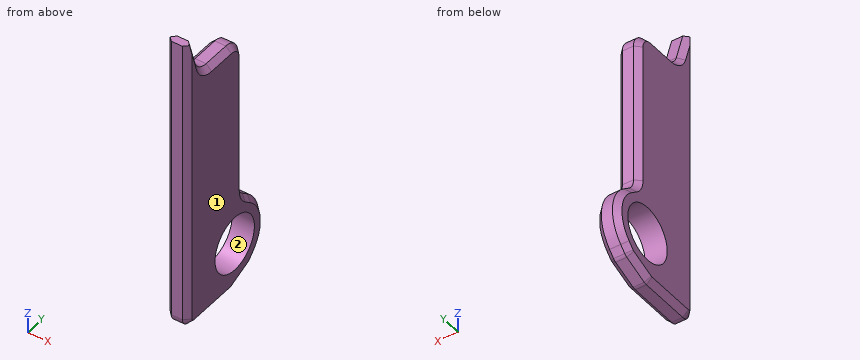
```python
from build123d import *

# Parameters (mm, degrees)
SKETCH_1_R      = 50
EXTRUDE_1_DEPTH = 40
FILLET_1_R      = 15
FILLET_2_R      = 15
CHAMFER_1_SIZE  = 10


with BuildPart() as part:
    # 草图1 → 凸台-拉伸1 (new body)
    with BuildSketch(Plane(origin=(0, 0, 0), x_dir=(0, 0, -1), z_dir=(1, 0, 0))):
        with BuildLine():
            Line((85, -8.5), (65, 41.5))
            Line((65, 41.5), (52.08314884, 53.966152419))
            ThreePointArc((52.08314884, 53.966152419), (-5.26193851, 74.815185645), (-59.124192044, 46.14466291))
            Line((-59.124192044, 46.14466291), (-69.350323182, 33.042134836))
            ThreePointArc((-69.350323182, 33.042134836), (-79.842035775, 24.539510808), (-93, 21.5))
            Line((-93, 21.5), (-348, 21.5))
            ThreePointArc((-348, 21.5), (-369.213203436, 12.713203436), (-378, -8.5))
            Line((-378, -8.5), (-378, -58.5))
            ThreePointArc((-378, -58.5), (-383.833102889, -76.275294204), (-399.064072268, -87.138247076))
            Line((-399.064072268, -87.138247076), (-451.500924593, -103.5))
            Line((-451.500924593, -103.5), (-451.500924593, -118.5))
            Line((-451.500924593, -118.5), (-116.500924593, -118.5))
            Line((-116.500924593, -118.5), (85, -118.5))
            Line((85, -118.5), (85, -8.5))
        make_face()
        Circle(SKETCH_1_R, mode=Mode.SUBTRACT)
    extrude(amount=EXTRUDE_1_DEPTH)

    # 圆角1
    fillet_1_edges = [part.edges().sort_by_distance(p)[0] for p in [
        (20, -118.5, -85),
    ]]
    fillet(fillet_1_edges, radius=FILLET_1_R)

    # 圆角2
    fillet_2_edges = [part.edges().sort_by_distance(p)[0] for p in [
        (20, 41.5, -65),
        (20, -8.5, -85),
    ]]
    fillet(fillet_2_edges, radius=FILLET_2_R)

    # 倒角1
    # the kernel refuses this chamfer: 10 mm, written as the material it takes off along each edge
    with BuildSketch(Plane(origin=(40, -118.5, -70), x_dir=(0.027495876610586317, 0.9996219169112968, 0), z_dir=(0, 0, 1))) as chamfer_1_piece_1:
        Polygon((CHAMFER_1_SIZE * 0.999621916911, CHAMFER_1_SIZE * 0.0274958766106), (-CHAMFER_1_SIZE * 0.0274958766106, CHAMFER_1_SIZE * 0.999621916911), (0, 0), align=None)
    extrude(amount=547.217754472, mode=Mode.SUBTRACT)
    with BuildSketch(Plane(origin=(0, -118.5, 477.217754472), x_dir=(0.9996219169112968, -0.027495876610586317, 0), z_dir=(0, 0, -1))) as chamfer_1_piece_2:
        Polygon((CHAMFER_1_SIZE * 0.999621916911, -CHAMFER_1_SIZE * 0.0274958766106), (-CHAMFER_1_SIZE * 0.0274958766106, -CHAMFER_1_SIZE * 0.999621916911), (0, 0), align=None)
    extrude(amount=547.217754472, mode=Mode.SUBTRACT)
    with BuildSketch(Plane(origin=(40, -87.138247076, 399.064072268), x_dir=(0.02749587661058635, -0.9542473146313191, -0.2977516402781551), z_dir=(0, -0.297864257716727, 0.9546082358616352)), Plane(origin=(0, -87.138247076, 399.064072268), x_dir=(0.9996219169112968, 0.026247790264700862, 0.008190038876882964), z_dir=(0, -0.297864257716727, 0.9546082358616352))) as chamfer_1_piece_3:
        Polygon((CHAMFER_1_SIZE * 0.999621916911, -CHAMFER_1_SIZE * 0.0274958766106), (-CHAMFER_1_SIZE * 0.0274958766106, -CHAMFER_1_SIZE * 0.999621916911), (0, 0), align=None)
    extrude(amount=80.647062361, mode=Mode.SUBTRACT)
    with BuildSketch(Plane(origin=(40, -58.5, 408), x_dir=(0, 0, -1), z_dir=(0, 1, 0))) as chamfer_1_piece_4:
        Polygon((30 + CHAMFER_1_SIZE, 0), (30, CHAMFER_1_SIZE), (30, 0), align=None)
    revolve(axis=Axis((40, -58.5, 408), (-1, 0, 0)), revolution_arc=72.670629443, mode=Mode.SUBTRACT)
    with BuildSketch(Plane(origin=(40, -8.5, 378), x_dir=(0.027495876610586282, 0, -0.9996219169112968), z_dir=(0, -1, 0)), Plane(origin=(0, -8.5, 378), x_dir=(0.9996219169112968, 0, 0.0274958766105877), z_dir=(0, -1, 0))) as chamfer_1_piece_5:
        Polygon((CHAMFER_1_SIZE * 0.999621916911, -CHAMFER_1_SIZE * 0.0274958766106), (-CHAMFER_1_SIZE * 0.0274958766106, -CHAMFER_1_SIZE * 0.999621916911), (0, 0), align=None)
    extrude(amount=50, mode=Mode.SUBTRACT)
    with BuildSketch(Plane(origin=(40, -8.5, 348), x_dir=(0, 1, 0), z_dir=(0, 0, -1))) as chamfer_1_piece_6:
        Polygon((30 - CHAMFER_1_SIZE, 0), (30, -CHAMFER_1_SIZE), (30, 0), align=None)
    revolve(axis=Axis((40, -8.5, 348), (1, 0, 0)), revolution_arc=90, mode=Mode.SUBTRACT)
    with BuildSketch(Plane(origin=(40, 21.5, 93), x_dir=(0.027495876610586317, -0.9996219169112968, 0), z_dir=(0, 0, 1)), Plane(origin=(0, 21.5, 93), x_dir=(0.9996219169112968, 0.027495876610586317, 0), z_dir=(0, 0, 1))) as chamfer_1_piece_7:
        Polygon((CHAMFER_1_SIZE * 0.999621916911, -CHAMFER_1_SIZE * 0.0274958766106), (-CHAMFER_1_SIZE * 0.0274958766106, -CHAMFER_1_SIZE * 0.999621916911), (0, 0), align=None)
    extrude(amount=255, mode=Mode.SUBTRACT)
    with BuildSketch(Plane(origin=(40, 51.5, 93), x_dir=(0, -0.6152621721387623, -0.7883225605899479), z_dir=(0, 0.7883225605899479, -0.6152621721387623))) as chamfer_1_piece_8:
        Polygon((30 + CHAMFER_1_SIZE, 0), (30, CHAMFER_1_SIZE), (30, 0), align=None)
    revolve(axis=Axis((40, 51.5, 93), (-1, 0, 0)), revolution_arc=52.029027347, mode=Mode.SUBTRACT)
    with BuildSketch(Plane(origin=(40, 46.14466291, 59.124192044), x_dir=(0.027495876610586327, -0.6150295519163572, -0.788024509161346), z_dir=(0, -0.7883225605899483, 0.6152621721387617)), Plane(origin=(0, 46.14466291, 59.124192044), x_dir=(0.9996219169112968, 0.016917172768288757, 0.021675619855322733), z_dir=(0, -0.7883225605899483, 0.6152621721387617))) as chamfer_1_piece_9:
        Polygon((CHAMFER_1_SIZE * 0.999621916911, -CHAMFER_1_SIZE * 0.0274958766106), (-CHAMFER_1_SIZE * 0.0274958766106, -CHAMFER_1_SIZE * 0.999621916911), (0, 0), align=None)
    extrude(amount=16.620770139, mode=Mode.SUBTRACT)
    with BuildSketch(Plane(origin=(40, 0, 0), x_dir=(0, 0.7195486989139618, -0.6944419845395472), z_dir=(0, -0.6944419845395472, -0.7195486989139618))) as chamfer_1_piece_10:
        Polygon((75 - CHAMFER_1_SIZE, 0), (75, -CHAMFER_1_SIZE), (75, 0), align=None)
    revolve(axis=Axis((40, 0, 0), (1, 0, 0)), revolution_arc=96.011794601, mode=Mode.SUBTRACT)
    with BuildSketch(Plane(origin=(40, 43.734636446, -62.684572962), x_dir=(0.027495876610586317, -0.7192766497194039, 0.6941794277691075), z_dir=(0, 0.6944419845395474, 0.7195486989139617)), Plane(origin=(0, 43.734636446, -62.684572962), x_dir=(0.9996219169112968, 0.019784622240646275, -0.019094291120110143), z_dir=(0, 0.6944419845395474, 0.7195486989139617))) as chamfer_1_piece_11:
        Polygon((CHAMFER_1_SIZE * 0.999621916911, -CHAMFER_1_SIZE * 0.0274958766106), (-CHAMFER_1_SIZE * 0.0274958766106, -CHAMFER_1_SIZE * 0.999621916911), (0, 0), align=None)
    extrude(amount=14.733435189, mode=Mode.SUBTRACT)
    with BuildSketch(Plane(origin=(40, 32.941405963, -52.267943193), x_dir=(0, 0.3713906763541047, -0.9284766908852589), z_dir=(0, -0.9284766908852589, -0.3713906763541047))) as chamfer_1_piece_12:
        Polygon((15 - CHAMFER_1_SIZE, 0), (15, -CHAMFER_1_SIZE), (15, 0), align=None)
    revolve(axis=Axis((40, 32.941405963, -52.267943193), (1, 0, 0)), revolution_arc=24.215823259, mode=Mode.SUBTRACT)
    with BuildSketch(Plane(origin=(40, -5.817875908, -83.927150363), x_dir=(0.027495876610586313, -0.37125025982007287, 0.9281256495501801), z_dir=(0, 0.9284766908852591, 0.37139067635410444)), Plane(origin=(0, -5.817875908, -83.927150363), x_dir=(0.9996219169112968, 0.010211712211354702, -0.025529280528386704), z_dir=(0, 0.9284766908852591, 0.37139067635410444))) as chamfer_1_piece_13:
        Polygon((CHAMFER_1_SIZE * 0.999621916911, -CHAMFER_1_SIZE * 0.0274958766106), (-CHAMFER_1_SIZE * 0.0274958766106, -CHAMFER_1_SIZE * 0.999621916911), (0, 0), align=None)
    extrude(amount=47.745024136, mode=Mode.SUBTRACT)
    with BuildSketch(Plane(origin=(40, -11.388736054, -70), x_dir=(0, 0, -1), z_dir=(0, -1, 0))) as chamfer_1_piece_14:
        Polygon((15 - CHAMFER_1_SIZE, 0), (15, -CHAMFER_1_SIZE), (15, 0), align=None)
    revolve(axis=Axis((40, -11.388736054, -70), (1, 0, 0)), revolution_arc=21.801409486, mode=Mode.SUBTRACT)
    with BuildSketch(Plane(origin=(40, -103.5, -85), x_dir=(0.027495876610586282, 0, 0.9996219169112968), z_dir=(0, 1, 0)), Plane(origin=(0, -103.5, -85), x_dir=(0.9996219169112968, 0, -0.027495876610586317), z_dir=(0, 1, 0))) as chamfer_1_piece_15:
        Polygon((CHAMFER_1_SIZE * 0.999621916911, -CHAMFER_1_SIZE * 0.0274958766106), (-CHAMFER_1_SIZE * 0.0274958766106, -CHAMFER_1_SIZE * 0.999621916911), (0, 0), align=None)
    extrude(amount=92.111263946, mode=Mode.SUBTRACT)
    with BuildSketch(Plane(origin=(40, -103.5, -70), x_dir=(0, -1, 0), z_dir=(0, 0, 1))) as chamfer_1_piece_16:
        Polygon((15 - CHAMFER_1_SIZE, 0), (15, -CHAMFER_1_SIZE), (15, 0), align=None)
    revolve(axis=Axis((40, -103.5, -70), (1, 0, 0)), revolution_arc=90, mode=Mode.SUBTRACT)
    with BuildSketch(Plane(origin=(0, -58.5, 408), x_dir=(0, 0, -1), z_dir=(0, 1, 0))) as chamfer_1_piece_17:
        Polygon((30, -CHAMFER_1_SIZE), (30 + CHAMFER_1_SIZE, 0), (30, 0), align=None)
    revolve(axis=Axis((0, -58.5, 408), (-1, 0, 0)), revolution_arc=72.670629443, mode=Mode.SUBTRACT)
    with BuildSketch(Plane(origin=(0, -8.5, 348), x_dir=(0, 1, 0), z_dir=(0, 0, -1))) as chamfer_1_piece_18:
        Polygon((30, CHAMFER_1_SIZE), (30 - CHAMFER_1_SIZE, 0), (30, 0), align=None)
    revolve(axis=Axis((0, -8.5, 348), (1, 0, 0)), revolution_arc=90, mode=Mode.SUBTRACT)
    with BuildSketch(Plane(origin=(0, 51.5, 93), x_dir=(0, -0.6152621721387623, -0.7883225605899479), z_dir=(0, 0.7883225605899479, -0.6152621721387623))) as chamfer_1_piece_19:
        Polygon((30, -CHAMFER_1_SIZE), (30 + CHAMFER_1_SIZE, 0), (30, 0), align=None)
    revolve(axis=Axis((0, 51.5, 93), (-1, 0, 0)), revolution_arc=52.029027347, mode=Mode.SUBTRACT)
    with BuildSketch(Plane(origin=(0, 0, 0), x_dir=(0, 0.7195486989139618, -0.6944419845395472), z_dir=(0, -0.6944419845395472, -0.7195486989139618))) as chamfer_1_piece_20:
        Polygon((75, CHAMFER_1_SIZE), (75 - CHAMFER_1_SIZE, 0), (75, 0), align=None)
    revolve(axis=Axis((0, 0, 0), (1, 0, 0)), revolution_arc=96.011794601, mode=Mode.SUBTRACT)
    with BuildSketch(Plane(origin=(0, 32.941405963, -52.267943193), x_dir=(0, 0.3713906763541047, -0.9284766908852589), z_dir=(0, -0.9284766908852589, -0.3713906763541047))) as chamfer_1_piece_21:
        Polygon((15, CHAMFER_1_SIZE), (15 - CHAMFER_1_SIZE, 0), (15, 0), align=None)
    revolve(axis=Axis((0, 32.941405963, -52.267943193), (1, 0, 0)), revolution_arc=24.215823259, mode=Mode.SUBTRACT)
    with BuildSketch(Plane(origin=(0, -11.388736054, -70), x_dir=(0, 0, -1), z_dir=(0, -1, 0))) as chamfer_1_piece_22:
        Polygon((15, CHAMFER_1_SIZE), (15 - CHAMFER_1_SIZE, 0), (15, 0), align=None)
    revolve(axis=Axis((0, -11.388736054, -70), (1, 0, 0)), revolution_arc=21.801409486, mode=Mode.SUBTRACT)
    with BuildSketch(Plane(origin=(0, -103.5, -70), x_dir=(0, -1, 0), z_dir=(0, 0, 1))) as chamfer_1_piece_23:
        Polygon((15, CHAMFER_1_SIZE), (15 - CHAMFER_1_SIZE, 0), (15, 0), align=None)
    revolve(axis=Axis((0, -103.5, -70), (1, 0, 0)), revolution_arc=90, mode=Mode.SUBTRACT)


solid = part.part
```
Work out the finished part from the listing and answer in its coordinate system (mm). Face numbers are marked on the shaded views. Give positions to 0.01 mm unless a question says otherwise; leave off trailing zeros. Loops run counter-clockwise (first coordinate to the right, second up) from the corner with the lowest first, then second, coordinate; pieces in that order, holes last. Notation, with made-up numbers: (3.5, 80.25) -> (18.5, 80.25) arc R23 ccw to (18.5, 105.25) -> close; hole circle Ø6 at (71, 77.25). An arc over 180 degrees is marked (long way). Write item = value, one per line. Start each with the question number.
(1) Find section D-D on z = 132.5. Give the vertices of the cut face in (x, y), and give its area (3 significant figures).
(2) Find section A-A on z = 0. Give the vertices of the cut face in (x, y), and give its area (3 significant figures).
(3) Find the intervals of material crossed by probe 1 along Y at (x, z) = (14.5, 0); probe 2 along Y at (x, z) = (15, 137); probe 3 along Z at (x, y) = (8.5, -27), in increasing order. Write a range as from..to.
(4) Find section C-C on y = -29.5. Give the vertices of the cut face in (x, z).
(5) Find section B-B on x = 22.5. Give the vertices of the cut face in (y, z).
(6) The mould has two halves that part along Z. Classify the marked faces 1 and 2: +Z half, -Z half, draft (parallel to the pull), parting line (faces both ways), or undercut.
(7) Given pin 1 Ø16 at (x, z) = (20, 178.5) entering from +Y; pin 2 Ø4 at (x, z) = (6, 303) entering from -Y; pin 3 Ø16 at (x, y) = (21, -41.5) entering from +Z, each flat-ended and moving along its own axis, determine where each tip first touches the part or whether it passes through.
From the geometry:
q1.outline = (0, -108.5) -> (10, -118.5) -> (30, -118.5) -> (40, -108.5) -> (40, 11.5) -> (30, 21.5) -> (10, 21.5) -> (0, 11.5) -> close
q1.area = 5,400 mm^2
q2.outline = (0, -108.5) -> (10, -118.5) -> (30, -118.5) -> (40, -108.5) -> (40, -50) -> (0, -50) -> close; (0, 50) -> (40, 50) -> (40, 65) -> (30, 75) -> (10, 75) -> (0, 65) -> close
q2.area = 3,540 mm^2
q3.probe_1 = -118.5..-50, 50..75
q3.probe_2 = -118.5..21.5
q3.probe_3 = -83.5..-42.08, 42.08..376.5
q4.outline = (0, -75) -> (10, -85) -> (30, -85) -> (40, -75) -> (40, -40.37) -> (0, -40.37) -> close; (0, 40.37) -> (40, 40.37) -> (40, 368) -> (30, 378) -> (10, 378) -> (0, 368) -> close
q5.outline = (-118.5, -70) arc R15 ccw to (-103.5, -85) -> (-11.39, -85) arc R15 ccw to (-5.82, -83.93) -> (38.51, -66.2) arc R15 ccw to (43.73, -62.68) -> (53.97, -52.08) arc R75 ccw to (46.14, 59.12) -> (33.04, 69.35) arc R30 cw to (21.5, 93) -> (21.5, 348) arc R30 ccw to (-8.5, 378) -> (-58.5, 378) arc R30 cw to (-87.14, 399.06) -> (-103.5, 451.5) -> (-118.5, 451.5) -> close; hole circle Ø100 at (0, 0)
q6.face_1 = draft
q6.face_2 = undercut
q7.pin_1 = 21.5
q7.pin_2 = -116.5
q7.pin_3 = 378
